Design review of the part built by this model. Coordinates are the model's own, in mm. Face numbers are marked on the shaded views. A direction names the side the tool comes from. Round coordinates to 2 decimals unless told otherwise and drop trailing zeros. Order: outer loops, then holes, each group sorted by start corner. A loop starts at its lowest first (then second) coordinate and runs counter-clockwise, first axis right, second up. Notation, with made-up numbers: (1.5, 55) - (44.5, 55) arc R29 cw to (44.5, 87) - close; hole circle Ø5 at (-34.75, -19). An arc over 180 degrees is marked (long way). Use CSV: the item, a comma, the result in double quotes.
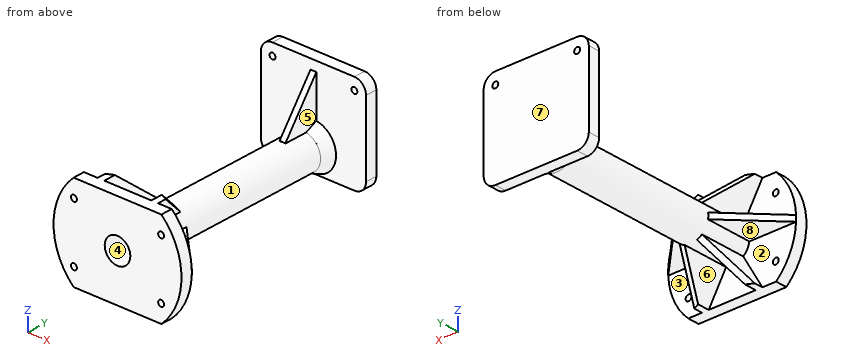
from build123d import *

# Parameters (mm, degrees)
SKETCH1_R                      = 2.55
SKETCH1_R_2                    = 11
BASE_DEPTH                     = 5
SKETCH1_3_R                    = 15
SKETCH1_3_R_2                  = 11
STEM_DEPTH                     = 200
SKETCH4_W                      = 90.4
SKETCH4_H                      = 40
TOP_PLATE_DEPTH                = 10
SKETCH6_W                      = 90.4
SKETCH6_H                      = 10
EXTRA_BACK_DEPTH               = 43.2
RIB1_START                     = -2.5
RIB1_DEPTH                     = 5
CUT_EXTRUDE1_REACH             = 217.059
SKETCH10_R                     = 2.55
CUT_EXTRUDE1_DIRECTION_2_DEPTH = 216.0592709
FILLET1_R                      = 10
FILLET2_R                      = 10
SKETCH11_R                     = 55
NEW_BASE_DEPTH                 = 10
RIB2_START                     = -2.5
RIB2_DEPTH                     = 5
CIRPATTERN7_COUNT              = 6
SKETCH13_R                     = 2.55
CUT_EXTRUDE2_DEPTH             = 10
FILLET3_R                      = 10
SKETCH15_R                     = 11
REMOVE_CENTER_DEPTH            = 208.65172766
BASE_CUT_DEPTH                 = 40
CHAMFER2_SIZE                  = 10
CHAMFER2_SIZE2                 = 4.452286853


with BuildPart() as part:
    # Sketch1 → base (new body)
    with BuildSketch(Plane(origin=(0, 0, 0), x_dir=(1, 0, 0), z_dir=(0, 1, 0))):
        with BuildLine():
            Line((-16, 25.377155081), (-42.833333333, 8.459051694))
            ThreePointArc((-42.833333333, 8.459051694), (-47.5, 0), (-42.833333333, -8.459051694))
            Line((-42.833333333, -8.459051694), (-16, -25.377155081))
            ThreePointArc((-16, -25.377155081), (0, -30), (16, -25.377155081))
            Line((16, -25.377155081), (42.833333333, -8.459051694))
            ThreePointArc((42.833333333, -8.459051694), (47.5, 0), (42.833333333, 8.459051694))
            Line((42.833333333, 8.459051694), (16, 25.377155081))
            ThreePointArc((16, 25.377155081), (0, 30), (-16, 25.377155081))
        make_face()
        with Locations(Location((-37.5, 0, 0), (0, 0, 270))):
            Circle(SKETCH1_R, mode=Mode.SUBTRACT)
        with Locations(Location((37.5, 0, 0), (0, 0, 270))):
            Circle(SKETCH1_R, mode=Mode.SUBTRACT)
        with Locations(Location((0, 0, 0), (0, 0, 270))):
            Circle(SKETCH1_R_2, mode=Mode.SUBTRACT)
    extrude(amount=BASE_DEPTH)

    # Sketch1<3> → stem (add)
    with BuildSketch(Plane(origin=(0, 0, 0), x_dir=(1, 0, 0), z_dir=(0, 1, 0))):
        with Locations(Location((0, 0, 0), (0, 0, 270))):
            Circle(SKETCH1_3_R)
        with Locations(Location((0, 0, 0), (0, 0, 270))):
            Circle(SKETCH1_3_R_2, mode=Mode.SUBTRACT)
    extrude(amount=STEM_DEPTH)

    # Sketch4 → top plate (add)
    with BuildSketch(Plane(origin=(0, 200, 0), x_dir=(1, 0, 0), z_dir=(0, 1, 0))):
        Rectangle(SKETCH4_W, SKETCH4_H)
    extrude(amount=-TOP_PLATE_DEPTH)

    # Sketch6 → extra back (add)
    with BuildSketch(Plane.XY.offset(20)):
        with Locations((0, 195)):
            Rectangle(SKETCH6_W, SKETCH6_H)
    extrude(amount=EXTRA_BACK_DEPTH)

    # Rib1: read off the stored shape, not the designer's step
    # Rib1 outline → Rib1 (add)
    with BuildSketch(Plane(origin=(0, 0, 0), x_dir=(0, 0, -1), z_dir=(1, 0, 0)).offset(RIB1_START)):
        Polygon((-15, 160), (-14.790199458, 160), (-14.790199458, 190), (-55, 190), align=None)
    extrude(amount=RIB1_DEPTH)

    # Sketch10 → Cut-Extrude1 (cut, up to next)
    with BuildSketch(Plane(origin=(0, 200, 0), x_dir=(1, 0, 0), z_dir=(0, 1, 0)), mode=Mode.PRIVATE) as cut_extrude1_sk1:
        with Locations(Location((35.2, -53.2, 0), (0, 0, 90))):
            Circle(SKETCH10_R)
    cut_extrude1_tool1 = extrude(cut_extrude1_sk1.sketch, amount=-CUT_EXTRUDE1_REACH, mode=Mode.PRIVATE) & part.part
    # Sketch10 → Cut-Extrude1 (cut, up to next)
    with BuildSketch(Plane(origin=(0, 200, 0), x_dir=(1, 0, 0), z_dir=(0, 1, 0)), mode=Mode.PRIVATE) as cut_extrude1_sk2:
        with Locations(Location((-35.2, -53.2, 0), (0, 0, 90))):
            Circle(SKETCH10_R)
    cut_extrude1_tool2 = extrude(cut_extrude1_sk2.sketch, amount=-CUT_EXTRUDE1_REACH, mode=Mode.PRIVATE) & part.part
    add(cut_extrude1_tool1.solids().sort_by_distance((35.2, 200, 53.2))[0], mode=Mode.SUBTRACT)
    add(cut_extrude1_tool2.solids().sort_by_distance((-35.2, 200, 53.2))[0], mode=Mode.SUBTRACT)

    # Sketch10 → Cut-Extrude1 direction 2 (cut)
    with BuildSketch(Plane(origin=(0, 200, 0), x_dir=(1, 0, 0), z_dir=(0, 1, 0))):
        with Locations(Location((35.2, -53.2, 0), (0, 0, 90))):
            Circle(SKETCH10_R)
        with Locations(Location((-35.2, -53.2, 0), (0, 0, 90))):
            Circle(SKETCH10_R)
    extrude(amount=CUT_EXTRUDE1_DIRECTION_2_DEPTH, mode=Mode.SUBTRACT)

    # Fillet1
    fillet1_edges = [part.edges().sort_by_distance(p)[0] for p in [
        (-45.2, 195, 63.2),
    ]]
    fillet(fillet1_edges, radius=FILLET1_R)

    # Fillet2
    fillet2_edges = [part.edges().sort_by_distance(p)[0] for p in [
        (45.2, 195, 63.2),
    ]]
    fillet(fillet2_edges, radius=FILLET2_R)

    # Sketch11 → new base (add)
    with BuildSketch(Plane.XZ):
        with Locations(Location((0, 0, 0), (0, 0, 270))):
            Circle(SKETCH11_R)
    extrude(amount=-NEW_BASE_DEPTH)

    # Rib2: read off the stored shape, not the designer's step
    # Rib2 outline → Rib2 (add)
    with BuildSketch(Plane.XY.offset(RIB2_START)):
        Polygon((13, 10), (55, 10), (13, 52), align=None)
    rib2 = extrude(amount=RIB2_DEPTH)

    # CirPattern7: Rib2 ×6 about axis
    cirpattern7_axis = Axis((0, 0, 0), (0, 1, 0))
    for i in range(1, CIRPATTERN7_COUNT):
        add(rib2.rotate(cirpattern7_axis, i * 360 / CIRPATTERN7_COUNT))

    # Sketch13 → Cut-Extrude2 (cut)
    with BuildSketch(Plane.XZ):
        with Locations(Location((-37.5, -25, 0), (0, 0, 270))):
            Circle(SKETCH13_R)
        with Locations(Location((-37.5, 25, 0), (0, 0, 270))):
            Circle(SKETCH13_R)
        with Locations(Location((37.5, 25, 0), (0, 0, 270))):
            Circle(SKETCH13_R)
        with Locations(Location((37.5, -25, 0), (0, 0, 270))):
            Circle(SKETCH13_R)
    extrude(amount=-CUT_EXTRUDE2_DEPTH, mode=Mode.SUBTRACT)

    # Fillet3
    fillet3_edges = [part.edges().sort_by_distance(p)[0] for p in [
        (45.2, 195, -20),
        (-45.2, 195, -20),
    ]]
    fillet(fillet3_edges, radius=FILLET3_R)

    # Sketch15 → remove center (cut, through all)
    with BuildSketch(Plane(origin=(0, 10, 0), x_dir=(1, 0, 0), z_dir=(0, 1, 0))):
        with Locations(Location((0, 0, 0), (0, 0, 270))):
            Circle(SKETCH15_R)
    extrude(amount=-REMOVE_CENTER_DEPTH, mode=Mode.SUBTRACT)

    # Sketch16 → base cut (cut)
    with BuildSketch(Plane.XZ):
        with BuildLine():
            Line((-37.749172176, 40), (37.749172176, 40))
            ThreePointArc((37.749172176, 40), (0, 55), (-37.749172176, 40))
        make_face()
        with BuildLine():
            ThreePointArc((-37.749172176, -40), (0, -55), (37.749172176, -40))
            Line((37.749172176, -40), (-37.749172176, -40))
        make_face()
    extrude(amount=-BASE_CUT_DEPTH, mode=Mode.SUBTRACT)


with BuildPart() as base_cut_kept_piece:
    # of the separate pieces the step leaves, the one the design keeps (base_cut_pieces_kept)
    add(part.part.solids().sort_by_distance((45.2, 190, -10))[0])

    # Chamfer2
    chamfer2_edges = [base_cut_kept_piece.edges().sort_by_distance(p)[0] for p in [
        (0, 190, -15),
    ]]
    chamfer2_side = [base_cut_kept_piece.faces().sort_by_distance(p)[0] for p in [
        (0, 100, -15),
    ]]
    chamfer(chamfer2_edges, length=CHAMFER2_SIZE, length2=CHAMFER2_SIZE2, reference=chamfer2_side[0])


solid = base_cut_kept_piece.part
1) We need section D-D (y = 101.5). Give the boundary of the cut face in (x, z), then the cut area to 3 significant figures.
Data:
outline,"circle Ø30 at (0, 0); hole circle Ø22 at (0, 0)"
area,"327 mm2"
2) For the marked faces 1, 2, 3, 4 and 5, list the 3-axis set-ups (+Z, -Z, +X, -X, +Y, -Y) from which the entire face can be reached by the end or side of a thin tool; tool diameter is ignored.
Data:
face 1,"none"
face 2,"-X"
face 3,"+X"
face 4,"-Y"
face 5,"+Z, +X"
3) The part is to be moulded in two halves that separate along Z. For the marked faces 6, 7 and 8, say which applies: +Z half, -Z half, draft (parallel to the pull), parting line (faces both ways), or undercut.
Data:
face 6,"-Z half"
face 7,"draft"
face 8,"undercut"
4) We need section C-C (z = 25). Give the boundary of the cut face in (x, y), then the cut area to 3 significant figures.
Data:
outline,"(-48.99, 0) - (-40.05, 0) - (-40.05, 10) - (-48.99, 10) - close; (-45.2, 190) - (-2.5, 190) - (-2.5, 167.5) - (2.5, 167.5) - (2.5, 190) - (45.2, 190) - (45.2, 200) - (-45.2, 200) - close; (-34.95, 0) - (34.95, 0) - (34.95, 10) - (17.32, 10) - (17.32, 34.69) - (11.55, 37.58) - (11.55, 10) - (-11.55, 10) - (-11.55, 37.58) - (-17.32, 34.69) - (-17.32, 10) - (-34.95, 10) - close; (40.05, 0) - (48.99, 0) - (48.99, 10) - (40.05, 10) - close"
area,"2,200 mm2"
5) We need section B-B (z = 36). Give the boundary of the cut face in (x, y), then the cut area to 3 significant figures.
Data:
outline,"(-45.2, 190) - (-2.5, 190) - (-2.5, 175.75) - (2.5, 175.75) - (2.5, 190) - (45.2, 190) - (45.2, 200) - (-45.2, 200) - close; (-41.58, 0) - (41.58, 0) - (41.58, 10) - (23.67, 10) - (23.67, 21.99) - (17.9, 24.87) - (17.9, 10) - (-17.9, 10) - (-17.9, 24.87) - (-23.67, 21.99) - (-23.67, 10) - (-41.58, 10) - close"
area,"1,960 mm2"
6) We need section A-A (x = -28). Give the boundary of the cut face in (y, z), then the cut area to 3 significant figures.
Data:
outline,"(0, -40) - (10, -40) - (10, -2.5) - (37, -2.5) - (37, 2.5) - (10, 2.5) - (10, 40) - (0, 40) - close; (190, -20) - (200, -20) - (200, 63.2) - (190, 63.2) - close"
area,"1,770 mm2"
7) Insertion check: pin 1 Ø6 at (x, z) = (-31, 13.5) entering from -Y; pin 2 Ø15 at (y, z) = (176, 31) entering from -X; pin 3 Ø11 at (x, z) = (1.5, -4) entering from -Y; pin 4 Ø5 at (y, z) = (98.5, 0.5) entering from +X. Each pin has a flat end and moves straight along its axis. Give the tip position at first contact, or say it passes through.
Data:
pin 1,"stops at y = 0"
pin 2,"stops at x = -2.5"
pin 3,"stops at y = 190"
pin 4,"stops at x = 15"
8) To check wall thickness, follow L1, parallel to Z at x = 37, y = 4; L2, parallel to Z at x = 0, y = 129; L3, parallel to X at y = 197.75, z = 53.2. State the ranges of each line that lie inside material, in increasing order. Write a range as from..to.
Data:
L1,"z = -40..-27.5, -22.5..22.5, 27.5..40"
L2,"z = -15..-11, 11..15"
L3,"x = -45.2..-37.75, -32.65..32.65, 37.75..45.2"
